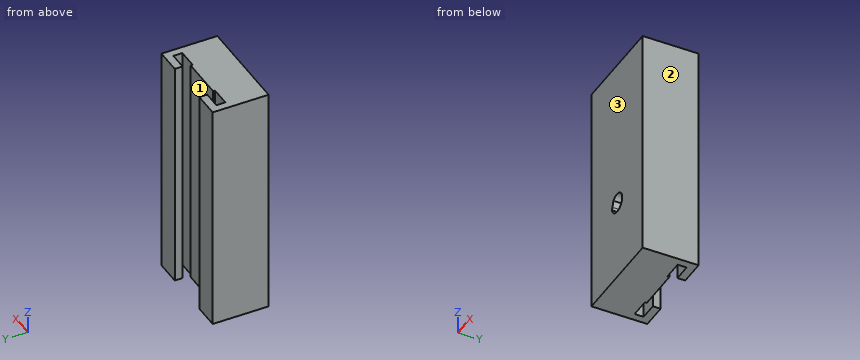
Autodesk Fusion 360 part; units mm, degrees
sketch "Sketch1" plane through (0, 0, 0) normal (0, 0, 1) x (1, 0, 0)
  line L0 (12.5, -5) -> (-12.5, -5)
  line L1 (-12.5, -5) -> (-12.5, 5)
  line L2 (12.5, 5) -> (12.5, -5)
  line L3 (12.5, -5) -> (-12.5, 5) construction
  line L4 (-12.5, -5) -> (12.5, 5) construction
  line L5 (12.5, 5) -> (12.5, 7.3)
  line L6 (10.5, 7.3) -> (10.5, 5)
  line L7 (-5.5, 5.5) -> (5.5, 5.5)
  line L8 (5.5, 5.5) -> (5.5, 5)
  line L9 (-5.5, 5) -> (-5.5, 5.5)
  line L10 (6, 9.3) -> (12.5, 9.3)
  line L11 (12.5, 9.3) -> (12.5, 7.3)
  line L12 (10.5, 7.3) -> (6, 7.3)
  line L13 (6, 7.3) -> (6, 9.3)
  line L14 (-10.5, 5) -> (-5.5, 5)
  line L15 (5.5, 5) -> (10.5, 5)
  line L16 (0, 5.5) -> (0, -5) construction
  line L17 (-6, 7.3) -> (-6, 9.3)
  line L18 (-12.5, 9.3) -> (-12.5, 7.3)
  line L19 (-10.5, 7.3) -> (-10.5, 5)
  line L20 (-12.5, 5) -> (-12.5, 7.3)
  line L21 (-10.5, 7.3) -> (-6, 7.3)
  line L22 (-6, 9.3) -> (-12.5, 9.3)
  dimension "d3" = 25
  dimension "d5" = 10
  dimension "d11" = 11
  dimension "d13" = 0.5
  dimension "d14" = 2.3
  dimension "d17" = 6.5
  dimension "d18" = 2
extrude "Extrude1" add sketch "Sketch1" along normal blind 30 and the other way blind 30
sketch "Sketch2" plane through (0, -5, 0) normal (0, -1, 0) x (1, 0, 0)
  line L0 (12.5, -30) -> (12.5, 30)
  line L1 (12.5, 30) -> (-12.5, 30)
  line L2 (-12.5, 30) -> (-12.5, -30)
  line L3 (-12.5, -30) -> (12.5, -30)
  circle A0 centre (0, 20) radius 9
  line L4 (0, 30) -> (0, 0) construction
  dimension "d23" = 18
extrude "Extrude2" cut sketch "Sketch2" against normal blind 5 contours A0
sketch "Sketch3" plane through (0, -5, 0) normal (0, -1, 0) x (1, 0, 0)
  circle A0 centre (0, 20) radius 9
  line L0 (12.5, -30) -> (12.5, 30)
  line L1 (12.5, 30) -> (-12.5, 30)
  line L2 (-12.5, 30) -> (-12.5, -30)
  line L3 (-12.5, -30) -> (12.5, -30)
  line L4 (0, 11) -> (0, -9) construction
  line L5 (2.3874, -9.7418) -> (8, -9.7418) construction
  line L6 (-2.2435, -8.7604) -> (-1.7674, -7.2318)
  line L7 (-2.2435, -8.7604) -> (-2.4588, -9.4519)
  arc A1 (-2.4588, -9.4519) -> (-1.7674, -7.2318) centre (0, -9) ccw
  point P0 (-9, 20)
  dimension "d26" = 5
extrude "Extrude3" cut sketch "Sketch3" against normal blind 7 contours L6 L7 A1
extrude "Extrude4" add 1 faces at (1.8705, 0, 22.3455) along direction (0, -1, 0) blind 5
Can you work these out from the model? Positions are in its coordinate system, mm. Face numbers are marked on the shaded views. Coordinates: 2 decimals unless noted, no trailing zeros. Write each loop counter-clockwise with the first axis right and the second up, starting at its lowest first coordinate (ties: lowest second). Pieces come first, ordered by that corner, then holes. Notation, with made-up numbers: (39.25, -32.75) - (89.25, -32.75) arc R28 cw to (89.25, -0.75) - close; hole circle Ø10 at (11.5, 7). An arc over 180 degrees is marked (long way). Return JSON: item names as keys, results as strings. Group by question number.
Item 1: We'd pull the mould along X, two halves only. Please class the marked faces 1, 2 and 3: pulls with the +X half, pulls with the -X half, needs draft (parallel to the pull), parting line crosses it, or undercut.
Item 2: If we section it at A-A (y = 8): Write out the boundary of the cut face in (x, z), then the cut area to 3 significant figures.
Item 3: If we section it at D-D (x = 1.25): Write out the boundary of the cut face in (y, z).
Item 4: Please list where these lines run through material, in increasing order: probe 1 along X at (y, z) = (6.25, -15.5); probe 2 along Y at (x, z) = (7.75, 22); probe 3 along X at (y, z) = (-0.75, -8.5).
Item 5: If we section it at C-C (z = 22): Write out the boundary of the cut face in (x, y).
Item 6: If we section it at B-B (x = -9.5): Write out the boundary of the cut face in (y, z).
Return value:
{
 "1": {"face 1": "undercut", "face 2": "pulls with the +X half", "face 3": "needs draft"},
 "2": {"outline": "(-12.5, -30) - (-6, -30) - (-6, 30) - (-12.5, 30) - close; (6, -30) - (12.5, -30) - (12.5, 30) - (6, 30) - close", "area": "780 mm^2"},
 "3": {"outline": "(-5, -30) - (5.5, -30) - (5.5, 30) - (-5, 30) - (-5, -6.83) - (2, -6.83) - (2, -11.17) - (-5, -11.17) - close"},
 "4": {"probe 1": "x = -12.5 to -10.5, 10.5 to 12.5", "probe 2": "y = -5 to 5, 7.3 to 9.3", "probe 3": "x = -12.5 to -2.16, 2.45 to 12.5"},
 "5": {"outline": "(-12.5, -5) - (12.5, -5) - (12.5, 9.3) - (6, 9.3) - (6, 7.3) - (10.5, 7.3) - (10.5, 5) - (5.5, 5) - (5.5, 5.5) - (-5.5, 5.5) - (-5.5, 5) - (-10.5, 5) - (-10.5, 7.3) - (-6, 7.3) - (-6, 9.3) - (-12.5, 9.3) - close"},
 "6": {"outline": "(-5, -30) - (5, -30) - (5, 30) - (-5, 30) - close; (7.3, -30) - (9.3, -30) - (9.3, 30) - (7.3, 30) - close"}
}
